Can you work these out from the model? Positions are in its coordinate system, mm. A direction names the side the tool comes from. Give positions to 0.01 mm unless a question says otherwise; leave off trailing zeros. Write each loop counter-clockwise with the first axis right and the second up, starting at its lowest first coordinate (ties: lowest second). Pieces come first, ordered by that corner, then holes. Notation, with made-up numbers: (24.5, 74) -> (46.5, 74) arc R24 ccw to (46.5, 86) -> close; hole circle Ø3 at (76.5, 41.5). An arc over 180 degrees is marked (long way). One line per item, written item: value.
from build123d import *

# Parameters (mm, degrees)
SKETCH_1_W      = 4
SKETCH_1_H      = 12
EXTRUDE_1_DEPTH = 4
FILLET_1_R      = 3


with BuildPart() as part:
    # ｽｹｯﾁ1 → ﾎﾞｽ - 押し出し1 (new body)
    with BuildSketch(Plane.XY):
        with BuildLine():
            Line((0, 2.5), (0, 5.5))
            Line((0, 5.5), (-15, 2.5))
            Line((-15, 2.5), (-15, -16))
            Line((-15, -16), (0, -16))
            Line((0, -16), (0, -2.5))
            ThreePointArc((0, -2.5), (-2.5, 0), (0, 2.5))
        make_face()
        with Locations((-10, -6)):
            Rectangle(SKETCH_1_W, SKETCH_1_H, mode=Mode.SUBTRACT)
    extrude(amount=EXTRUDE_1_DEPTH)

    # ﾌｨﾚｯﾄ1
    fillet_1_edges = [part.edges().sort_by_distance(p)[0] for p in [
        (-15, -16, 2),
        (-15, 2.5, 2),
    ]]
    fillet(fillet_1_edges, radius=FILLET_1_R)


solid = part.part
1) Will this pin go through, and if not, where does the flat tip stop? pin 1 (1 mm diameter, centred on x = -13, z = 3, fed in from -Y).
Answer list:
pin 1: stops at y = -15.96
2) We'd pull the mould along X, two halves only. Please class faces 3 (the face through (-7.6, -7.5, 0)), 4 (the face through (-15, -6, 2)), 5 (the face through (-10, -12, 2)): released by +X, released by -X, zero draft, split by the parting line, or undercut.
Answer list:
face 3: zero draft
face 4: released by -X
face 5: undercut
3) If we section it at B-B (y = -9.5): Write out the boundary of the cut face in (x, z), and give its area (3 significant figures).
Answer list:
outline: (-15, 0) -> (-12, 0) -> (-12, 4) -> (-15, 4) -> close; (-8, 0) -> (0, 0) -> (0, 4) -> (-8, 4) -> close
area: 44.0 mm^2
4) For faces 1 (the face through (-8, -6, 2)), 2 (the face through (-14.14, -15.1, 2.03)), which set-ups out of +Z, -Z, +X, -X, +Y, -Y let a thin tool reach every point of the face, with its end or its side?
Answer list:
face 1: +Z, -Z
face 2: +Z, -Z, -X, -Y
5) If we section it at D-D (y = 4.25): Write out the boundary of the cut face in (x, z), and give its area (3 significant figures).
Answer list:
outline: (-6.25, 0) -> (0, 0) -> (0, 4) -> (-6.25, 4) -> close
area: 25.0 mm^2
6) I need wall thicknesses on L1, parallel to X at y = -7.75, z = 3.2; L2, parallel to Y at x = -2.25, z = 3.45; L3, parallel to Y at x = -10.5, z = 3.4. Which ranges of each line are inside material? Lowest first, please.
Answer list:
L1: x = -15 to -12, -8 to 0
L2: y = -16 to -1.09, 1.09 to 5.05
L3: y = -16 to -12, 0 to 3.4
7) If we section it at A-A (x = -9.5): Write out the boundary of the cut face in (y, z), and give its area (3 significant figures).
Answer list:
outline: (-16, 0) -> (-12, 0) -> (-12, 4) -> (-16, 4) -> close; (0, 0) -> (3.6, 0) -> (3.6, 4) -> (0, 4) -> close
area: 30.4 mm^2
8) If we section it at C-C (z = 0.7): Write out the boundary of the cut face in (x, y).
Answer list:
outline: (-15, -13) arc R3 ccw to (-12, -16) -> (0, -16) -> (0, -2.5) arc R2.5 cw to (0, 2.5) -> (0, 5.5) -> (-12.59, 2.98) arc R3 ccw to (-15, 0.04) -> close; hole (-12, -12) -> (-8, -12) -> (-8, 0) -> (-12, 0) -> close
